Input: part model. Units: mm. Frame: model coordinates. A direction names the side the tool comes from. Coordinates: 2 decimals unless noted, no trailing zeros. Write each loop counter-clockwise with the first axis right and the second up, starting at its lowest first coordinate (ties: lowest second). Pieces come first, ordered by that corner, then holes. Notation, with made-up numbers: (46, 84) - (78, 84) arc R24 ccw to (78, 99) - close; hole circle Ø11 at (85, 84.25). An arc over 180 degrees is marked (long way). One line per question, with ' | ' between items. Start each with the question number.
1) First-contact query: P1, Ø1.2, axis at x = -9, y = 0.5, coming from the +Z side; P2, Ø8, axis at y = 9.5, z = -54.5, coming from the +X side; P3, Ø1.6, axis at y = 3, z = -14, coming from the -X side. Flat tips, straight axial feed; report the tip coordinate or a pass-through.
2) Draft query along X for faces 1 (the flat face through (0.6, 3, -12)), 2 (the cylindrical face through (-2.23, 12.79, -4.03)), 3 (the flat face through (-13, 15, -2.875)). Return one class per face: released by +X, released by -X, zero draft, split by the parting line, or undercut.
3) Line query: line 1 (Z direction, x = -3.5, y = 12.75) (3 decimals); line 2 (X direction, y = 12.8, z = -61.5) (3 decimals); line 3 (Z direction, x = -0.5, y = 2.5). Output: solid intervals per line, ascending.
4) Section query D-D on y = 10.5. Return loops of the section in (x, z).
5) Reachability of faces 4 (the cylindrical face through (-0.91, 12.81, -64.05)), 5 (the flat face through (-9, 15, -56.925)), 6 (the flat face through (0.304, 2.079, -7.395)), 7 (the flat face through (-1, 14, -32)) from +Z, -Z, +X, -X, +Y, -Y: full face, straight path, thin tool, end or side. Return the list, or none.
6) Section query B-B on z = -28.5. Return loops of the section in (x, y).
7) Section query C-C on x = -26. Return loops of the section in (y, z).
8) Section query A-A on x = -17.5. Return loops of the section in (y, z) (3 decimals).
Autodesk Inventor part; units mm, degrees
ref_plane "YZ Plane" through (0, 0, 0) normal (1, 0, 0) x (0, 1, 0)
ref_plane "XZ Plane" through (0, 0, 0) normal (0, 1, 0) x (-1, 0, 0)
ref_plane "XY Plane" through (0, 0, 0) normal (0, 0, 1) x (1, 0, 0)
sketch "Sketch1" plane through (0, 0, 0) normal (0, 1, 0) x (-1, 0, 0)
  line L0 (0, 0) -> (30, 0)
  line L1 (30, 0) -> (30, -65)
  line L2 (30, -65) -> (0, -65)
  line L3 (0, -65) -> (0, 0)
  circle A0 centre (26.5, -3.5) radius 1.375
  circle A1 centre (3.5, -3.5) radius 1.375
  circle A2 centre (26.5, -61.5) radius 1.375
  circle A3 centre (3.5, -61.5) radius 1.375
  line L4 (15, 0) -> (15, -65)
  line L5 (30, -32.5) -> (0, -32.5)
  dimension "d0" = 65
  dimension "d1" = 30
  dimension "d2" = 3.5
  dimension "d3" = 3.5
  dimension "d4" = 3.5
  dimension "d5" = 3.5
  dimension "d6" = 3.5
  dimension "d7" = 3.5
  dimension "d8" = 3.5
  dimension "d9" = 3.5
  dimension "d10" = 2.75
  dimension "d11" = 2.75
  dimension "d12" = 2.75
  dimension "d13" = 2.75
  dimension "d14" = 15
  dimension "d15" = 32.5
extrude "Extrusion1" add sketch "Sketch1" along normal blind 1.5
fillet "Fillet1" radius 3 4 edges at (-30, 0.75, 0) (0, 0.75, 0) (0, 0.75, -65) (-30, 0.75, -65)
sketch "Sketch2" plane through (0, 1.5, 0) normal (0, 1, 0) x (1, 0, 0)
  line L0 (-6.9, 6.8) -> (0.6, 6.8)
  line L1 (0.6, 6.8) -> (0.6, 18)
  line L2 (0.6, 18) -> (-6.9, 18)
  line L3 (-6.9, 18) -> (-6.9, 6.8)
  line L4 (-27, 0) -> (-3, 0)
  line L5 (-15, 0) -> (-15, 64.9233)
  line L6 (-30, 62) -> (-30, 3)
  line L7 (0.6, 12.4) -> (-6.9, 12.4)
  line L8 (-4.1, 57.95) -> (1.4, 57.95)
  line L9 (1.4, 57.95) -> (1.4, 50.05)
  line L10 (1.4, 50.05) -> (-4.1, 50.05)
  line L11 (-4.1, 50.05) -> (-4.1, 57.95)
  line L12 (-4.1, 45.35) -> (1.4, 45.35)
  line L13 (1.4, 45.35) -> (1.4, 37.45)
  line L14 (1.4, 37.45) -> (-4.1, 37.45)
  line L15 (-4.1, 37.45) -> (-4.1, 45.35)
  line L16 (-4.1, 41.4) -> (1.4, 41.4)
  line L17 (-4.1, 54) -> (1.4, 54)
  line L18 (-22.4, 12.8) -> (-11.4, 12.8)
  line L19 (-11.4, 12.8) -> (-11.4, -2.6)
  line L20 (-11.4, -2.6) -> (-22.4, -2.6)
  line L21 (-22.4, -2.6) -> (-22.4, 12.8)
  line L22 (-16.9, 12.8) -> (-16.9, -2.6)
  line L23 (0, 3) -> (0, 62)
  line L24 (-23.5, 65.9) -> (-6.5, 65.9)
  line L25 (-6.5, 65.9) -> (-6.5, 61.9)
  line L26 (-6.5, 61.9) -> (-23.5, 61.9)
  line L27 (-23.5, 61.9) -> (-23.5, 65.9)
  line L28 (-15, 65.9) -> (-15, 61.9)
  point P0 (0, 0)
  dimension "d19" = 11.2
  dimension "d20" = 7.5
  dimension "d21" = 15
  dimension "d23" = 12.4
  dimension "d24" = 7.9
  dimension "d25" = 7.9
  dimension "d26" = 5.5
  dimension "d27" = 3.95
  dimension "d28" = 3.95
  dimension "d29" = 41.4
  dimension "d30" = 54
  dimension "d32" = 30.6
  dimension "d33" = 31.4
  dimension "d34" = 11
  dimension "d35" = 15.4
  dimension "d36" = 2.6
  dimension "d37" = 5.5
  dimension "d38" = 16.9
  dimension "d39" = 65.9
  dimension "d40" = 4
  dimension "d41" = 17
  dimension "d42" = 8.5
  dimension "d43" = 15
extrude "Extrusion2" add sketch "Sketch2" along normal blind 3.25 contours L3 L7 L23 L0 | L23 L7 L1 L0 | L3 L2 L23 L7 | L23 L2 L1 L7
extrude "Extrusion3" add sketch "Sketch2" along normal blind 2.55 contours L10 L11 L17 L23 | L23 L17 L9 L10 | L14 L15 L16 L23 | L23 L16 L13 L14 | L23 L12 L13 L16 | L16 L15 L12 L23 | L23 L8 L9 L17 | L17 L11 L8 L23
extrude "Extrusion4" add sketch "Sketch2" along normal blind 1.25 contours L26 L27 L24 L28 L5 | L5 L28 L24 L25 L26
extrude "Extrusion5" add sketch "Sketch2" along normal blind 1.35 contours L21 L18 L22 L4 | L4 L22 L20 L21 | L22 L18 L5 L4 | L4 L19 L20 L22 | L5 L18 L19 L4
sketch "Sketch3" plane through (0, 1.5, 0) normal (0, 1, 0) x (1, 0, 0)
  line L0 (-29, 6.95) -> (-24, 6.95)
  line L1 (-24, 6.95) -> (-24, 58.05)
  line L2 (-24, 58.05) -> (-29, 58.05)
  line L3 (-29, 58.05) -> (-29, 6.95)
  line L4 (-26.5, 58.05) -> (-26.5, 6.95)
  circle A0 centre (-26.5, 3.5) radius 1.375
  line L5 (-26.5, 3.5) -> (-26.5, 61.8145)
  line L6 (-27, 0) -> (-22.4, 0)
  point P0 (0, 0)
  dimension "d52" = 5
  dimension "d53" = 6.95
  dimension "d54" = 51.1
extrude "Extrusion6" add sketch "Sketch3" along normal blind 10.5 contours L3 L2 L4 L0 | L4 L2 L1 L0
chamfer "Chamfer1" distance 1.1735 angle 45 2 edges at (0.3, 1.5, -6.8) (0.3, 1.5, -18)
chamfer "Chamfer2" distance 0.889 angle 45 4 edges at (0.7, 1.5, -37.45) (0.7, 1.5, -45.35) (0.7, 1.5, -50.05) (0.7, 1.5, -57.95)
sketch "Sketch4" plane through (0, 12, 0) normal (0, 1, 0) x (1, 0, 0)
  line L0 (0, 0) -> (-30, 0)
  line L1 (-30, 0) -> (-30, 65)
  line L2 (-30, 65) -> (0, 65)
  line L3 (0, 65) -> (0, 0)
  circle A0 centre (-26.5, 3.5) radius 1.375
  circle A1 centre (-26.5, 3.5) radius 1.375
  circle A2 centre (-3.5, 3.5) radius 1.375
  circle A3 centre (-3.5, 61.5) radius 1.375
  circle A4 centre (-26.5, 61.5) radius 1.375
  dimension "d63" = 30
  dimension "d64" = 65
  dimension "d67" = 3.5
  dimension "d68" = 3.5
  dimension "d69" = 3.5
  dimension "d70" = 3.5
  dimension "d71" = 3.5
  dimension "d72" = 3.5
  dimension "d73" = 3.5
  dimension "d74" = 3.5
extrude "Extrusion7" add sketch "Sketch4" along normal blind 1.6 contours L0 L1 L2 L3 | A0 | A2 | A3 | A4
extrude "Extrusion8" cut sketch "Sketch4" along normal blind 2 contours A0 | A2 | A3 | A4
fillet "Fillet2" radius 3.175 4 edges at (-30, 12.8, 0) (0, 12.8, 0) (0, 12.8, -65) (-30, 12.8, -65)
sketch "Sketch5" plane through (0, 13.6, 0) normal (0, 1, 0) x (1, 0, 0)
  line L0 (-18.875, 64.265) -> (-12.625, 64.265)
  line L1 (-12.625, 64.265) -> (-12.625, 57.915)
  line L2 (-12.625, 57.915) -> (-18.875, 57.915)
  line L3 (-18.875, 57.915) -> (-18.875, 64.265)
  line L4 (-12.396, 56.925) -> (-6.146, 56.925)
  line L5 (-6.146, 56.925) -> (-6.146, 50.575)
  line L6 (-6.146, 50.575) -> (-12.396, 50.575)
  line L7 (-12.396, 50.575) -> (-12.396, 56.925)
  line L8 (-18.61, 13.125) -> (-8.31, 13.125)
  line L9 (-8.31, 13.125) -> (-8.31, 2.875)
  line L10 (-8.31, 2.875) -> (-18.61, 2.875)
  line L11 (-18.61, 2.875) -> (-18.61, 13.125)
  line L12 (-18.875, 57.915) -> (-12.625, 64.265) construction
  line L13 (-18.875, 64.265) -> (-12.625, 57.915) construction
  line L14 (-18.61, 2.875) -> (-8.31, 13.125) construction
  line L15 (-18.61, 13.125) -> (-8.31, 2.875) construction
  line L16 (-26.825, 0) -> (-3.175, 0) construction
  line L17 (0, 3.175) -> (0, 61.825) construction
  line L18 (-12.396, 50.575) -> (-6.146, 56.925) construction
  line L19 (-12.396, 56.925) -> (-6.146, 50.575) construction
  line L20 (-3.175, 65) -> (-26.825, 65) construction
  line L21 (-30, 61.825) -> (-30, 3.175) construction
  line L22 (-24, 15.26) -> (-1, 15.26)
  line L23 (-1, 15.26) -> (-1, 49.76)
  line L24 (-1, 49.76) -> (-24, 49.76)
  line L25 (-24, 49.76) -> (-24, 15.26)
  line L26 (-24, 15.26) -> (-1, 49.76) construction
  line L27 (-24, 49.76) -> (-1, 15.26) construction
  point P0 (0, 0)
  point P1 (-13.46, 8)
  point P2 (-9.271, 53.75)
  point P3 (-15.75, 61.09)
  point P4 (-12.5, 32.51)
  dimension "d80" = 6.35
  dimension "d81" = 6.25
  dimension "d82" = 6.25
  dimension "d83" = 6.35
  dimension "d84" = 10.3
  dimension "d85" = 10.25
  dimension "d87" = 8
  dimension "d88" = 13.46
  dimension "d90" = 9.271
  dimension "d91" = 15.75
  dimension "d94" = 3.91
  dimension "d95" = 11.25
  dimension "d98" = 6
  dimension "d99" = 23
  dimension "d100" = 34.5
  dimension "d101" = 32.51
extrude "Extrusion9" add sketch "Sketch5" along normal blind 2.3 contours L0 L1 L2 L3 | L4 L5 L6 L7
extrude "Extrusion10" add sketch "Sketch5" along normal blind 3.6 contours L8 L9 L10 L11
extrude "Extrusion11" add sketch "Sketch5" along normal blind 1.7 contours L25 L24 L23 L22
equation "\"d11\" = d10"
equation "\"d12\" = d10"
equation "\"d13\" = d10"
equation "\"d14\" = 0.5 * d1"
equation "\"d15\" = 0.5 * d0"
equation "\"d21\" = d14"
equation "\"d25\" = d24"
equation "\"d27\" = 0.5 * d25"
equation "\"d37\" = 0.5 * d34"
equation "\"d42\" = 0.5 * d41"
equation "\"d43\" = d14"
equation "\"d53\" = -0.5 * d54 + 0.5 * d0"
equation "\"d83\" = d80"
properties part number "pizero_model" material "UHMW, Black"
Answer key:
1) P1: z = 0 | P2: x = 0 | P3: x = -29
2) face 1: released by +X | face 2: undercut | face 3: zero draft
3) line 1: -65 to -62.875, -60.125 to -4.875, -2.125 to 0 | line 2: -30 to -27.875, -25.125 to -4.875, -2.125 to 0 | line 3: -57.95 to -50.05, -45.35 to -37.45, -18 to -6.8
4) outline: (-29, -58.05) - (-24, -58.05) - (-24, -6.95) - (-29, -6.95) - close
5) face 4: -Z, +X, +Y | face 5: -Z, +X, -X, +Y | face 6: +Z, +X, -Y | face 7: +Z, -Z, +X, +Y
6) outline: (-30, 0) - (0, 0) - (0, 1.5) - (-24, 1.5) - (-24, 12) - (0, 12) - (0, 13.6) - (-1, 13.6) - (-1, 15.3) - (-24, 15.3) - (-24, 13.6) - (-30, 13.6) - (-30, 12) - (-29, 12) - (-29, 1.5) - (-30, 1.5) - close
7) outline: (0, -65) - (1.5, -65) - (1.5, -62.78) - (0, -62.78) - close; (0, -60.22) - (1.5, -60.22) - (1.5, -58.05) - (12, -58.05) - (12, -60.22) - (13.6, -60.22) - (13.6, -4.78) - (12, -4.78) - (12, -6.95) - (1.5, -6.95) - (1.5, -4.78) - (0, -4.78) - close; (0, -2.22) - (1.5, -2.22) - (1.5, 0) - (0, 0) - close; (12, -65) - (13.6, -65) - (13.6, -62.78) - (12, -62.78) - close; (12, -2.22) - (13.6, -2.22) - (13.6, 0) - (12, 0) - close
8) outline: (0, -65) - (1.5, -65) - (1.5, -65.9) - (2.75, -65.9) - (2.75, -61.9) - (1.5, -61.9) - (1.5, -12.8) - (2.85, -12.8) - (2.85, 2.6) - (1.5, 2.6) - (1.5, 0) - (0, 0) - close; (12, -65) - (13.6, -65) - (13.6, -64.265) - (15.9, -64.265) - (15.9, -57.915) - (13.6, -57.915) - (13.6, -49.76) - (15.3, -49.76) - (15.3, -15.26) - (13.6, -15.26) - (13.6, -13.125) - (17.2, -13.125) - (17.2, -2.875) - (13.6, -2.875) - (13.6, 0) - (12, 0) - close
